Input: part model. Units: mm. Frame: model coordinates. A direction names the side the tool comes from. Coordinates: 2 decimals unless noted, no trailing zeros. Loops run counter-clockwise (first coordinate to the right, second up) from the corner with the lowest first, then second, coordinate; pieces in that order, holes last. Notation, with made-up numbers: M 33,13.5 L 40,13.5 A17 ccw 40,38.5 Z; hole C 7.25,17.25 d2. An arc over 180 degrees is marked long. Use a Markdown table: item, result. Add a question column.
1. Pin query (flat end, axial travel): pin 1 (2 mm diameter, centred on x = -3.5, z = 5.5, fed in from +Y); pin 2 (3.5 mm diameter, centred on x = 2.5, y = 0.5, fed in from +Z); pin 3 (2 mm diameter, centred on y = 2, z = 31, fed in from -X); pin 4 (4.5 mm diameter, centred on x = 0, y = 0, fed in from +Z). Return the tip coordinate at first contact, or that it passes through.
2. Draft query along X for faces 1 (the flat face through (-5.226, 2.938, 18.802)), 2 (the flat face through (4.1, -1.3, 27.9)), 3 (the flat face through (-8, 10, 38.7)). Return one class per face: +X half, -X half, draft (parallel to the pull), parting line (faces both ways), or undercut.
3. Section B-B on z = 7. Output: boundary loops of the cut face in (x, y), then the cut area to 3 significant figures.
4. Section A-A on z = 27. Output: boundary loops of the cut face in (x, y), then the cut area to 3 significant figures.
5. Set-up query: faces 4 (the flat face through (5.226, -2.938, 18.802)), 5 (the flat face through (-3.48, 1.96, 20.8)), 6 (the cylindrical face through (1.071, -8.154, 28.722)). Return all of +Z, -Z, +X, -X, +Y, -Y with unobstructed straight access to the full face (end or side cutting, diameter ignored); none if empty.
6. Line query: L1, parallel to Y at x = 0, z = 9; L2, parallel to Y at x = 0, z = 30.4; L3, parallel to X at y = -1.5, z = 12. Output: solid intervals per line, ascending. Write a range as [from, to].
```python
from build123d import *

# Parameters (mm, degrees)
SKETCH1_R           = 5.95
BOSS_EXTRUDE1_DEPTH = 11.9
M6_TAPPED_HOLE1_D   = 5
BOSS_EXTRUDE2_DEPTH = 14
CHAMFER1_SIZE       = 0.5
SHELL1_START        = 13.9
SHELL1_DEPTH        = 24.8
SHELL1_START_2      = 27.9
SHELL1_2_OUTLINE_R  = 6.224211325
SHELL1_2_DEPTH      = 10.8
SKETCH6_R           = 2.5
CUT_EXTRUDE1_DEPTH  = 35.179526035


with BuildPart() as part:
    # Sketch1 → Boss-Extrude1 (new body)
    with BuildSketch(Plane.XY):
        Circle(SKETCH1_R)
    extrude(amount=BOSS_EXTRUDE1_DEPTH)

    # M6 Tapped Hole1 (through all)
    with Locations(Plane(origin=(0, 0, 0), x_dir=(-1, 0, 0), z_dir=(0, 0, -1))):
        with Locations((0, 0)):
            Hole(M6_TAPPED_HOLE1_D / 2)

    # Sketch4 → Boss-Extrude2 (add)
    with BuildSketch(Plane.XY.offset(11.9)):
        Polygon((6.921331173, 0.134625435), (3.34407654, 6.061361341), (-3.577254633, 5.926735906), (-6.921331173, -0.134625435), (-3.34407654, -6.061361341), (3.577254633, -5.926735906), align=None)
    extrude(amount=BOSS_EXTRUDE2_DEPTH)

    # Sketch5 → Revolve1 (revolve)
    with BuildSketch(Plane(origin=(0, 0, 0), x_dir=(1, 0, 0), z_dir=(0, 1, 0))):
        with BuildLine():
            Line((-6.921331173, -25.9), (-8.224211325, -25.9))
            Line((-8.224211325, -25.9), (-8.224211325, -31.466244152))
            ThreePointArc((-8.224211325, -31.466244152), (-8.886011508, -33.819165828), (-10.677341595, -35.48210191))
            Line((-10.677341595, -35.48210191), (-15, -37.7))
            Line((-15, -37.7), (-15, -38.7))
            Line((-15, -38.7), (0, -38.7))
            Line((0, -38.7), (0, -25.9))
            Line((0, -25.9), (-6.921331173, -25.9))
        make_face()
    revolve(axis=Axis((0, 0, 0), (0, 0, 1)))

    # Chamfer1
    chamfer1_edges = [part.edges().sort_by_distance(p)[0] for p in [
        (-5.95, 0, 0),
    ]]
    chamfer(chamfer1_edges, length=CHAMFER1_SIZE)

    # Shell1: read off the stored shape, not the designer's step
    # Shell1 outline → Shell1 (cut)
    with BuildSketch(Plane.XY.offset(SHELL1_START)):
        Polygon((-2.228488616, -4.039283965), (2.383878219, -3.949569736), (4.612366834, 0.089714229), (2.228488616, 4.039283965), (-2.383878219, 3.949569736), (-4.612366834, -0.089714229), align=None)
    extrude(amount=SHELL1_DEPTH, mode=Mode.SUBTRACT)

    # Shell1 2 outline → Shell1 2 (cut)
    with BuildSketch(Plane.XY.offset(SHELL1_START_2)):
        Circle(SHELL1_2_OUTLINE_R)
        Polygon((4.612366834, 0.089714229), (2.383878219, -3.949569736), (-2.228488616, -4.039283965), (-4.612366834, -0.089714229), (-2.383878219, 3.949569736), (2.228488616, 4.039283965), align=None, mode=Mode.SUBTRACT)
    extrude(amount=SHELL1_2_DEPTH, mode=Mode.SUBTRACT)

    # Shell1 3 outline → Shell1 3 (revolve, cut)
    with BuildSketch(Plane.XZ):
        with BuildLine():
            ThreePointArc((6.224211325, 31.466244152), (7.179257815, 34.861754834), (9.764333429, 37.261544544))
            Line((9.764333429, 37.261544544), (12.567866916, 38.7))
            Line((12.567866916, 38.7), (6.224211325, 38.7))
            Line((6.224211325, 38.7), (6.224211325, 31.466244152))
        make_face()
    revolve(axis=Axis((0, 0, 0), (0, 0, 1)), mode=Mode.SUBTRACT)

    # Sketch6 → Cut-Extrude1 (cut, through all)
    with BuildSketch(Plane(origin=(0, 0, 11.9), x_dir=(-1, 0, 0), z_dir=(0, 0, -1))):
        Circle(SKETCH6_R)
    extrude(amount=-CUT_EXTRUDE1_DEPTH, mode=Mode.SUBTRACT)


solid = part.part
```
Answers below:
| question | item | result |
|---|---|---|
| 1 | pin 1 | stops at y = 5.4 |
| 1 | pin 2 | stops at z = 27.9 |
| 1 | pin 3 | stops at x = -8.16 |
| 1 | pin 4 | passes through |
| 2 | face 1 | -X half |
| 2 | face 2 | undercut |
| 2 | face 3 | draft |
| 3 | outline | C 0,0 d11.9; hole C 0,0 d5 |
| 3 | area | 91.6 mm² |
| 4 | outline | C 0,0 d16.45; hole M -4.61,-0.09 L -2.23,-4.04 L 2.38,-3.95 L 4.61,0.09 L 2.23,4.04 L -2.38,3.95 Z |
| 4 | area | 157 mm² |
| 5 | face 4 | -Z, +X, -Y |
| 5 | face 5 | +Z |
| 5 | face 6 | -Z |
| 6 | L1 | y = [-5.95, -2.5], [2.5, 5.95] |
| 6 | L2 | y = [-8.22, -6.22], [6.22, 8.22] |
| 6 | L3 | x = [-6.1, -2], [2, 6.02] |
